Read the model definition and answer for the solid it produces. Units are mm, in the model's axes. Face numbers are marked on the shaded views. A direction names the side the tool comes from. Coordinates: 2 decimals unless noted, no trailing zeros. Write each loop counter-clockwise with the first axis right and the second up, starting at its lowest first coordinate (ties: lowest second). Pieces come first, ordered by that corner, then holes.
(1) The part is cut by section D-D, the plane x = 33. Determine the outline of the cut face in (y, z).
(2) Given pin 1 (12 mm diameter, centred on x = -22, z = 48.5, fed in from -Y); pin 2 (2.5 mm diameter, centred on x = 0.5, z = 29.5, fed in from -Y); pin 3 (5 mm diameter, centred on y = -46, z = 29.5, fed in from -X), each flat-ended and moving along its own axis, determine where each tip first touches the part or whether it passes through.
(3) Determine the mould class of the marked faces 4, 5, 6 and 7 for opening direction Z: pulls with the +Z half, pulls with the -Z half, needs draft (parallel to the pull), parting line crosses it, or undercut.
(4) The part is cut by section B-B, the plane y = -9.5. Determine the outline of the cut face in (x, z), and give its area (3 significant figures).
(5) Which of the six approach directions +Z, -Z, +X, -X, +Y, -Y give full straight-line access (tool end or side, diameter ignored) to the marked faces 1, 2 and 3?
(6) The part is cut by section A-A, the plane x = -25. Determine the outline of the cut face in (y, z), and give its area (3 significant figures).
(7) Straight lines are drawn through the part: line 1 along X through (y, z) = (-28.5, 22); line 2 along Y through (x, z) = (-25, 39.5); line 3 along X through (y, z) = (-42, 56). For each, find the intervals that lie inside material, in ascending order.
(8) The part is cut by section C-C, the plane z = 49.5. Determine the outline of the cut face in (x, y), and give its area (3 significant figures).
Autodesk Fusion 360 part; units mm, degrees
sketch "Sketch1" plane through (0, 0, 0) normal (0, 0, 1) x (1, 0, 0) in component "Box"
  line L0 (-43.441, -63.6961) -> (52.559, -63.6961)
  line L1 (52.559, -63.6961) -> (52.559, 0.3039)
  line L2 (52.559, 0.3039) -> (-43.441, 0.3039)
  line L3 (-43.441, 0.3039) -> (-43.441, -63.6961)
  line L4 (-43.441, -15.6961) -> (52.559, -15.6961)
  line L5 (-163.441, -63.6961) -> (36.559, -63.6961)
  line L6 (36.559, -63.6961) -> (36.559, -43.6961)
  line L7 (36.559, -43.6961) -> (-163.441, -43.6961)
  line L8 (-163.441, -43.6961) -> (-163.441, -63.6961)
  circle A0 centre (16.559, -43.6961) radius 12
  line L9 (36.559, -43.6961) -> (36.559, -15.6961)
  line L10 (-3.441, -63.6961) -> (-3.441, -15.6961)
  line L11 (-3.441, -43.6961) -> (-43.441, -15.6961)
  dimension "d1" = 96
  dimension "d2" = 64
  dimension "d3" = 16
  dimension "d4" = 200
  dimension "d5" = 20
  dimension "d6" = 16
  dimension "d7" = 24
  dimension "d8" = 20
  dimension "d9" = 20
  dimension "d10" = 40
  dimension "d11" = 28
  dimension "d12" = 40
extrude "Extrude1" add sketch "Sketch1" along normal blind 12 contours L4 L10 L11 in component "Box"
extrude "Extrude2" add sketch "Sketch1" along normal blind 42 contours L4 L7 A0 L9 L10 in component "Box"
sketch "Sketch2" plane through (0, 0, 0) normal (0, 0, 1) x (1, 0, 0) in component "Box"
  line L0 (36.559, -16.6004) -> (36.559, 0)
  line L1 (52.559, -63.6961) -> (52.559, 0.3039)
  dimension "d17" = 16
extrude "Extrude3" add sketch "Sketch1" along normal blind 64 contours L0 L1 L4 L6 L9 in component "Box"
sketch "Sketch3" plane through (0, -63.6961, 0) normal (0, -1, 0) x (1, 0, 0) in component "Box"
  line L0 (36.559, 0) -> (52.559, 0)
  line L1 (52.559, 0) -> (52.559, 64)
  line L2 (52.559, 64) -> (36.559, 64)
  line L3 (36.559, 64) -> (36.559, 0)
sketch "Sketch4" plane through (0, -43.6961, 0) normal (0, -1, 0) x (1, 0, 0) in component "Box"
  line L0 (28.559, 0) -> (36.559, 0)
  line L1 (36.559, 0) -> (36.559, 42)
  line L2 (36.559, 42) -> (28.559, 42)
  line L3 (28.559, 42) -> (28.559, 0)
  line L4 (52.3937, 32) -> (52.3937, 0) construction
  dimension "d20" = 32
sketch "Sketch5" plane through (52.559, 0, 0) normal (1, 0, 0) x (0, 1, 0) in component "Box"
  line L0 (-63.6961, 0) -> (-15.6961, 0)
  line L1 (-15.6961, 0) -> (-15.6961, 64)
  line L2 (-15.6961, 64) -> (-63.6961, 64) construction
  line L3 (-63.6961, 64) -> (-63.6961, 0)
  arc A0 (-31.6961, 64) -> (-63.6953, 32) centre (-31.6953, 32) ccw
  line L4 (-31.6953, 32) -> (69.344, 47.5915) construction
  line L5 (-63.6961, 34.0454) -> (-63.6961, 29.5) construction
  point P0 (18.8244, 39.7958)
  dimension "d24" = 32
  dimension "d25" = 32
  dimension "d28" = 16
sketch "Sketch6" plane through (52.559, 0, 0) normal (1, 0, 0) x (0, 1, 0) in component "Box"
  line L0 (-63.6961, 0) -> (-15.6961, 0)
  line L1 (-15.6961, 0) -> (-15.6961, 64)
  line L2 (-15.6961, 64) -> (-63.6961, 64)
  line L3 (-63.6961, 64) -> (-63.6961, 0)
sketch "Sketch7" plane through (52.559, -39.6961, 32) normal (1, 0, 0) x (0, 1, 0) in component "Box"
  arc A0 (7.6874, 74.9842) -> (-66.58, -0.2294) centre (8.2336, 0.1714) ccw
  arc A1 (8, 32.1706) -> (7.6874, 74.9842) centre (7.8437, 53.5774) ccw
  arc A2 (8, 32.1706) -> (-23.7659, 0) centre (8.2336, 0.1714) ccw
  arc A3 (-66.58, -0.2294) -> (-23.7659, 0) centre (-45.173, -0.1147) ccw
  arc A4 (7.8437, 53.5774) -> (-45.173, -0.1147) centre (8.2336, 0.1714) ccw construction
  line L0 (24, -32) -> (24, 32)
  line L1 (-24, -32) -> (40, -32)
  dimension "d29" = 32
  dimension "d30" = 16
  dimension "d31" = 32
extrude "Extrude4" cut sketch "Sketch7" against normal blind 30 in component "Box"
sketch "Sketch8" plane through (0, 0, 0) normal (1, 0, 0) x (0, 1, 0) in component "Box"
  line L0 (-63.6961, 0) -> (0.3039, 0)
  point P0 (-63.6953, 32)
  dimension "d34" = 32
extrude "Extrude5" add sketch "Sketch1" along normal blind 64 contours L1 L2 L3 L4 in component "Box"
sketch "Sketch9" plane through (0, 0, 0) normal (0, 0, 1) x (1, 0, 0) in component "Box"
  line L0 (52.559, 0.3039) -> (-43.441, 0.3039)
  point P0 (52.559, -31.6961)
  dimension "d37" = 32
sketch "Sketch10" plane through (0, -15.6961, 0) normal (0, -1, 0) x (1, 0, 0) in component "Box"
  line L0 (36.559, 42) -> (36.559, 64)
  line L1 (36.559, 64) -> (-43.441, 64)
  line L2 (-43.441, 64) -> (-43.441, 12)
  line L3 (-43.441, 12) -> (-3.441, 12)
  line L4 (-3.441, 12) -> (-3.441, 42)
  line L5 (-3.441, 42) -> (36.559, 42)
  line L6 (-43.441, 64) -> (-43.441, 28.223) construction
  line L7 (-43.441, 28.223) -> (-8.4006, 28.223) construction
  circle A0 centre (-23.441, 28.223) radius 8
  line L8 (-23.441, 28.223) -> (-23.441, 48.1368) construction
  line L9 (-23.441, 48.1368) -> (-23.441, 12.9343) construction
  line L10 (-23.441, 20.223) -> (-43.441, 20.223)
  line L11 (-43.441, 20.223) -> (-43.441, 36.223)
  line L12 (-43.441, 36.223) -> (-23.441, 36.223)
  line L13 (-23.441, 36.223) -> (-23.441, 20.223)
  dimension "d38" = 35.777
  dimension "d39" = 16
  dimension "d40" = 20
  dimension "d41" = 20
  dimension "d42" = 16
extrude "Extrude6" cut sketch "Sketch10" against normal blind 155 contours L2 A0 L10 L11 L12 | A0 L13 | A0 L13 in component "Box"
component "Box" placed x (1, 0, 0) y (0, 1, 0) z (0, 0, 1) at (0, 0, 0)
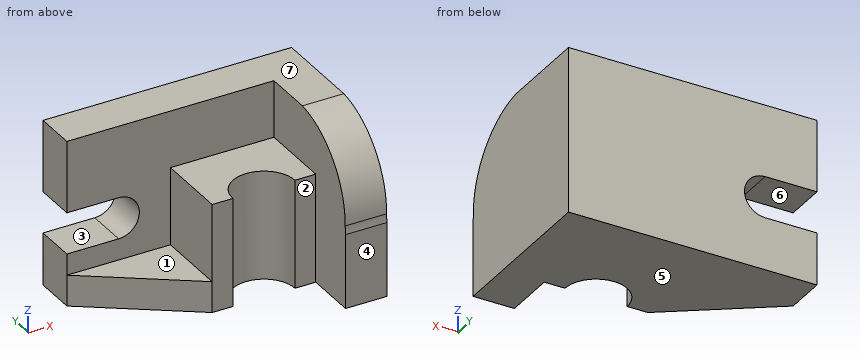
Computed:
1. outline: (-43.7, 0) - (0.3, 0) - (0.3, 64) - (-15.7, 64) - (-15.7, 42) - (-43.7, 42) - close
2. pin 1: stops at y = -15.7
2. pin 2: stops at y = -43.7
2. pin 3: stops at x = -3.44
3. face 4: needs draft
3. face 5: pulls with the -Z half
3. face 6: undercut
3. face 7: pulls with the +Z half
4. outline: (-43.44, 0) - (52.56, 0) - (52.56, 64) - (-43.44, 64) - (-43.44, 36.22) - (-23.44, 36.22) arc R8 cw to (-23.44, 20.22) - (-43.44, 20.22) - close
4. area: 5,720 mm2
5. face 1: +Z, -X, -Y
5. face 2: +Z, -Z, -X, -Y
5. face 3: -X, +Y, -Y
6. outline: (-28.6, 0) - (0.3, 0) - (0.3, 20.22) - (-15.7, 20.22) - (-15.7, 12) - (-28.6, 12) - close; (-15.7, 36.22) - (0.3, 36.22) - (0.3, 64) - (-15.7, 64) - close
6. area: 923 mm2
7. line 1: x = -3.44 to 52.56
7. line 2: y = -15.7 to 0.3
7. line 3: x = 36.56 to 52.56
8. outline: (-43.44, -15.7) - (36.56, -15.7) - (36.56, -58.36) - (52.56, -58.36) - (52.56, 0.3) - (-43.44, 0.3) - close
8. area: 2,220 mm2
